The listing builds one solid part. Answer for the finished solid, in the listing's coordinates (mm). A direction names the side the tool comes from. Give positions to 0.01 mm unless a question says otherwise; leave off trailing zeros. Loops run counter-clockwise (first coordinate to the right, second up) from the corner with the lowest first, then second, coordinate; pieces in that order, holes last. Notation, with made-up numbers: (59.25, -39.75) - (106.25, -39.75) arc R6 cw to (106.25, -34.75) - close; hole circle Ø6 at (-18.5, 43.25). An arc over 180 degrees is marked (long way). Answer in a Markdown table with one row per item. Add a question column.
```python
from build123d import *

# Parameters (mm, degrees)
BOSS_EXTRUDE1_DEPTH = 14
CUT_EXTRUDE1_DEPTH  = 28.51465704
CHAMFER1_SIZE       = 1
FILLET1_R           = 2
SKETCH3_R           = 1.75
CUT_EXTRUDE2_DEPTH  = 26.403494878
SKETCH4_R           = 1.7
CUT_EXTRUDE3_DEPTH  = 36.01151742
SKETCH5_R           = 3
CUT_EXTRUDE4_DEPTH  = 3
CUT_EXTRUDE5_DEPTH  = 3


with BuildPart() as part:
    # Sketch1 → Boss-Extrude1 (new body)
    with BuildSketch(Plane(origin=(0, 0, 0), x_dir=(1, 0, 0), z_dir=(0, 1, 0))):
        Polygon((-12.5, 0), (12.5, 0), (12.5, -3), (6, -3), (6, -20.1198), (-6, -20.1198), (-6, -3), (-12.5, -3), align=None)
    extrude(amount=BOSS_EXTRUDE1_DEPTH)

    # Sketch2 → Cut-Extrude1 (cut, through all)
    with BuildSketch(Plane(origin=(0, 14, 0), x_dir=(1, 0, 0), z_dir=(0, 1, 0))):
        with BuildLine():
            Line((-0.5, -12.119769411), (-0.5, -20.1198))
            Line((-0.5, -20.1198), (0.5, -20.1198))
            Line((0.5, -20.1198), (0.5, -12.119769411))
            ThreePointArc((0.5, -12.119769411), (0, -3.85), (-0.5, -12.119769411))
        make_face()
    extrude(amount=-CUT_EXTRUDE1_DEPTH, mode=Mode.SUBTRACT)

    # Chamfer1
    chamfer1_edges = [part.edges().sort_by_distance(p)[0] for p in [
        (0, 0, 3.85),
        (0, 14, 3.85),
    ]]
    chamfer(chamfer1_edges, length=CHAMFER1_SIZE)

    # Fillet1
    fillet1_edges = [part.edges().sort_by_distance(p)[0] for p in [
        (-12.5, 0, 1.5),
        (6, 7, 20.1198),
        (-6, 7, 20.1198),
        (12.5, 14, 1.5),
        (-12.5, 14, 1.5),
        (12.5, 0, 1.5),
    ]]
    fillet(fillet1_edges, radius=FILLET1_R)

    # Sketch3 → Cut-Extrude2 (cut, through all)
    with BuildSketch(Plane.XY.offset(3)):
        with Locations((-9.5, 11)):
            Circle(SKETCH3_R)
        with Locations((9.5, 11)):
            Circle(SKETCH3_R)
    extrude(amount=-CUT_EXTRUDE2_DEPTH, mode=Mode.SUBTRACT)

    # Sketch4 → Cut-Extrude3 (cut, through all)
    with BuildSketch(Plane(origin=(12.5, 0, 0), x_dir=(0, 0, -1), z_dir=(1, 0, 0))):
        with Locations((-15.5, 7)):
            Circle(SKETCH4_R)
        with BuildLine():
            Line((-2, 0), (-2, 4.5))
            ThreePointArc((-2, 4.5), (-1.414213562, 5.914213562), (0, 6.5))
            Line((0, 6.5), (0, 0))
            Line((0, 0), (-2, 0))
        make_face()
    extrude(amount=-CUT_EXTRUDE3_DEPTH, mode=Mode.SUBTRACT)

    # Sketch5 → Cut-Extrude4 (cut)
    with BuildSketch(Plane(origin=(6, 0, 0), x_dir=(0, 0, -1), z_dir=(1, 0, 0))):
        with Locations((-15.5, 7)):
            Circle(SKETCH5_R)
    extrude(amount=-CUT_EXTRUDE4_DEPTH, mode=Mode.SUBTRACT)

    # Sketch6 → Cut-Extrude5 (cut)
    with BuildSketch(Plane.ZY.offset(6)):
        Polygon((15.5, 3.535898385), (18.5, 5.267949192), (18.5, 8.732050808), (15.5, 10.464101615), (12.5, 8.732050808), (12.5, 5.267949192), align=None)
    extrude(amount=-CUT_EXTRUDE5_DEPTH, mode=Mode.SUBTRACT)


solid = part.part
```
(1) A cutting plane is placed at D-D on z = 15. Determine the outline of the cut face in (x, y), plus the area to 3 significant figures.
(2) A tool of negligible diameter and unlimited length cuts with its end or side. For faces 4 (the face through (6, 7, 10)), 5 (the face through (-5.4, 7.1, 19.55)), 6 (the face through (0.184, 0.84, 3.694)), 7 (the face through (-0.5, 9, 16)), 8 (the face through (-4.5, 9.6, 17)), from which of +Z, -Z, +X, -X, +Y, -Y can it reach the whole face along a straight path? Write none if from no direction.
(3) A cutting plane is placed at A-A on x = 9.5. Determine the outline of the cut face in (y, z).
(4) A cutting plane is placed at C-C on y = 11. Determine the outline of the cut face in (x, z).
(5) Given pin 1 Ø1.5 at (x, y) = (7, 3.5) entering from +Z; pin 2 Ø3 at (y, z) = (6.5, 7) entering from -X; pin 3 Ø2 at (x, y) = (-9.5, 11) entering from +Z; pin 4 Ø1.5 at (x, y) = (-5, 7.5) entering from +Z, each flat-ended and moving along its own axis, determine where each tip first touches the part or whether it passes through.
(6) Find the intervals of material crossed by line 1 along X through (y, z) = (11, 14.75); line 2 along X through (y, z) = (8.25, 16.75); line 3 along Y through (x, z) = (1.8, 15.5), in increasing order. Write a range as [from, to].
(7) The mould has two halves that part along Z. Classify faces 1 (the face through (-11.9, 0.57, 2.49)), 2 (the face through (-4.5, 4.4, 14)), 3 (the face through (0, 2, 2)): pulls with the +Z half, pulls with the -Z half, needs draft (parallel to the pull), parting line crosses it, or undercut.
(8) A cutting plane is placed at B-B on z = 8. Determine the outline of the cut face in (x, y), plus the area to 3 significant figures.
Evaluation:
| question | item | result |
|---|---|---|
| 1 | outline | (-6, 0) - (-0.5, 0) - (-0.5, 5.38) - (-3, 5.38) - (-3, 3.82) - (-6, 3.82) - close; (-6, 10.18) - (-3, 10.18) - (-3, 8.62) - (-0.5, 8.62) - (-0.5, 14) - (-6, 14) - close; (0.5, 0) - (6, 0) - (6, 4.04) - (3, 4.04) - (3, 5.38) - (0.5, 5.38) - close; (0.5, 8.62) - (3, 8.62) - (3, 9.96) - (6, 9.96) - (6, 14) - (0.5, 14) - close |
| 1 | area | 101 mm² |
| 2 | face 4 | +Z, +X, +Y, -Y |
| 2 | face 5 | +Z, -X, +Y, -Y |
| 2 | face 6 | -Y |
| 2 | face 7 | +Z, +Y, -Y |
| 2 | face 8 | -X |
| 3 | outline | (0, 2) - (4.5, 2) arc R2 cw to (6.5, 0) - (9.25, 0) - (9.25, 3) - (0, 3) - close; (12.75, 0) - (14, 0) - (14, 3) - (12.75, 3) - close |
| 4 | outline | (-12.5, 0) - (-11.25, 0) - (-11.25, 3) - (-12.5, 3) - close; (-7.75, 0) - (7.75, 0) - (7.75, 3) - (6, 3) - (6, 18.12) arc R2 ccw to (4, 20.12) - (0.5, 20.12) - (0.5, 12.12) arc R4.15 cw (long way) to (-0.5, 12.12) - (-0.5, 20.12) - (-4, 20.12) arc R2 ccw to (-6, 18.12) - (-6, 3) - (-7.75, 3) - close; (11.25, 0) - (12.5, 0) - (12.5, 3) - (11.25, 3) - close |
| 5 | pin 1 | stops at z = 3 |
| 5 | pin 2 | stops at x = -6 |
| 5 | pin 3 | passes through |
| 5 | pin 4 | stops at z = 20.1 |
| 6 | line 1 | x = [-6, -0.5], [0.5, 6] |
| 6 | line 2 | x = [-3, -0.5], [0.5, 3] |
| 6 | line 3 | y = [0, 5.3], [8.7, 14] |
| 7 | face 1 | needs draft |
| 7 | face 2 | undercut |
| 7 | face 3 | pulls with the -Z half |
| 8 | outline | (-6, 0) - (-5.15, 0) - (-4.15, 1) - (-4.15, 13) - (-5.15, 14) - (-6, 14) - close; (4.15, 1) - (5.15, 0) - (6, 0) - (6, 14) - (5.15, 14) - (4.15, 13) - close |
| 8 | area | 49.8 mm² |
